Verification items for this drawing (mm, ordinates from the low corner). A direction names the side the tool comes from. Round coordinates to 2 decimals unless told otherwise and drop trailing zeros. Order: outer loops, then holes, each group sorted by start corner. A loop starts at its lowest first (then second) coordinate and runs counter-clockwise, first axis right, second up. Notation, with made-up numbers: (-17, 19.5) - (17, 19.5) arc R25 ccw to (17, 51.5) - close; hole circle Ø6 at (37, 34). An arc over 180 degrees is marked (long way). Use a Markdown table: item, result. Add a question column.
(1) Access from +Z, -Z, +X, -X, +Y, -Y to the whole of each face (thin tool, end or side, straight path). Record for the marked faces 4, 5, 6 and 7.
(2) Section check D-D on x = 20.5. Record the boundary of the cut face in (y, z), then the cut area to 3 significant figures.
(3) Section check A-A on x = 5. Record the boundary of the cut face in (y, z).
(4) Section check C-C on y = 6.5. Record the boundary of the cut face in (x, z), then the cut area to 3 significant figures.
(5) Mould release check, pull along Z, two halves, no side actions. Record for the marked faces 1, 2 and 3: released by +Z, released by -Z, zero draft, split by the parting line, or undercut.
(6) Thickness scan on line 1 along X through (y, z) = (40.9, 5); line 2 along X through (y, z) = (32, 25.5); line 3 along Z through (x, y) = (26.5, 37.5). Record the ranges inside material, lowest first. Write a range as [from, to].
(7) Gauge pin test, flat ends, axial feed: P1, Ø5, axis at x = 5, z = 5, coming from the -Y side; P2, Ø12, axis at y = 22, z = 38.5, coming from the -X side; P3, Ø5, axis at x = 23.5, y = 20.5, coming from the -Z side; P4, Ø20, axis at x = 27, y = 27, coming from the +Z side. Record the tip position at first contact, or that the pin passes through.
(8) Section check B-B on z = 5. Record the boundary of the cut face in (x, y).
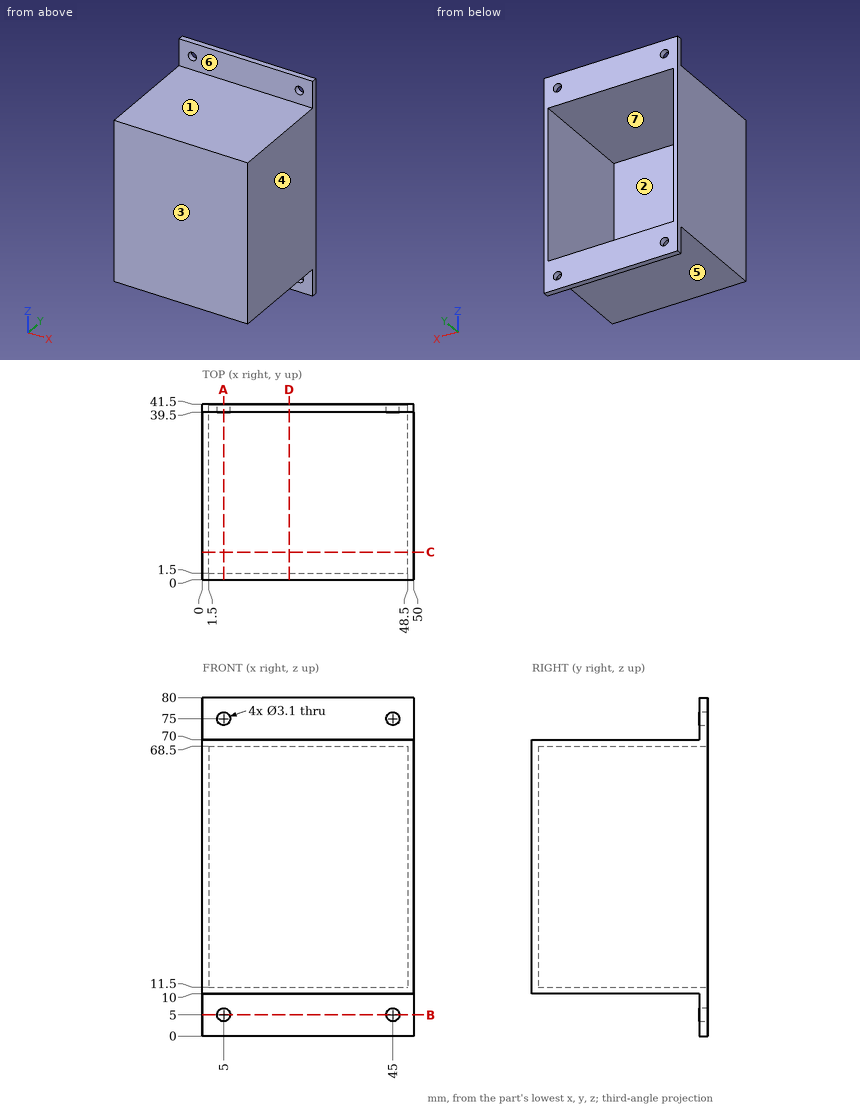
Check sheet entries:
| question | item | result |
|---|---|---|
| 1 | face 4 | +Z, -Z, +X, +Y, -Y |
| 1 | face 5 | -Z, +X, -X, -Y |
| 1 | face 6 | +Z, +X, -X, -Y |
| 1 | face 7 | +Y |
| 2 | outline | (0, 10) - (39.5, 10) - (39.5, 0) - (41.5, 0) - (41.5, 11.5) - (1.5, 11.5) - (1.5, 68.5) - (41.5, 68.5) - (41.5, 80) - (39.5, 80) - (39.5, 70) - (0, 70) - close |
| 2 | area | 250 mm2 |
| 3 | outline | (0, 10) - (39.5, 10) - (39.5, 6.55) - (41.5, 6.55) - (41.5, 11.5) - (1.5, 11.5) - (1.5, 68.5) - (41.5, 68.5) - (41.5, 73.45) - (39.5, 73.45) - (39.5, 70) - (0, 70) - close; (39.5, 0) - (41.5, 0) - (41.5, 3.45) - (39.5, 3.45) - close; (39.5, 76.55) - (41.5, 76.55) - (41.5, 80) - (39.5, 80) - close |
| 4 | outline | (0, 10) - (50, 10) - (50, 70) - (0, 70) - close; hole (1.5, 11.5) - (48.5, 11.5) - (48.5, 68.5) - (1.5, 68.5) - close |
| 4 | area | 321 mm2 |
| 5 | face 1 | released by +Z |
| 5 | face 2 | undercut |
| 5 | face 3 | zero draft |
| 6 | line 1 | x = [0, 3.45], [6.55, 43.45], [46.55, 50] |
| 6 | line 2 | x = [0, 1.5], [48.5, 50] |
| 6 | line 3 | z = [10, 11.5], [68.5, 70] |
| 7 | P1 | stops at y = 39.5 |
| 7 | P2 | stops at x = 0 |
| 7 | P3 | stops at z = 10 |
| 7 | P4 | stops at z = 70 |
| 8 | outline | (0, 39.5) - (3.45, 39.5) - (3.45, 41.5) - (0, 41.5) - close; (6.55, 39.5) - (43.45, 39.5) - (43.45, 41.5) - (6.55, 41.5) - close; (46.55, 39.5) - (50, 39.5) - (50, 41.5) - (46.55, 41.5) - close |
